from build123d import *

# Parameters (mm, degrees)
SKETCH1_R           = 1
BOSS_EXTRUDE1_DEPTH = 2.95
CUT_EXTRUDE1_DEPTH  = 0.5
SKETCH3_R           = 0.75
BOSS_EXTRUDE2_DEPTH = 3
FILLET1_R           = 0.5


with BuildPart() as part:
    # Sketch1 → Boss-Extrude1 (new body, symmetric)
    with BuildSketch(Plane(origin=(0, 0, 0), x_dir=(1, 0, 0), z_dir=(0, 1, 0))):
        Polygon((-6.5, -3.1), (-5, -3.1), (-4.5, -3.6), (-2.5, -3.6), (-2, -3.1), (2, -3.1), (2.5, -3.6), (4.5, -3.6), (5, -3.1), (6.5, -3.1), (6.5, 3.1), (5.9, 3.1), (-7.417700692, 5.9), (-7.5, 5.50855802), (3.955876716, 3.1), (-6.5, 3.1), align=None)
        with Locations((3.5, -1.9)):
            Circle(SKETCH1_R, mode=Mode.SUBTRACT)
        with Locations((-3.5, -1.9)):
            Circle(SKETCH1_R, mode=Mode.SUBTRACT)
    extrude(amount=BOSS_EXTRUDE1_DEPTH, both=True)

    # Sketch2 → Cut-Extrude1 (cut)
    with BuildSketch(Plane(origin=(0, 2.95, 0), x_dir=(1, 0, 0), z_dir=(0, 1, 0))):
        Polygon((5.9, 3.1), (3.955876716, 3.1), (-7.5, 5.50855802), (-7.417700692, 5.9), align=None)
    cut_extrude1 = extrude(amount=-CUT_EXTRUDE1_DEPTH, mode=Mode.SUBTRACT)

    # Mirror1: Cut-Extrude1 across plane
    add(cut_extrude1.mirror(Plane.ZX), mode=Mode.SUBTRACT)

    # Sketch3 → Boss-Extrude2 (add)
    with BuildSketch(Plane.XY.offset(3.1)):
        Circle(SKETCH3_R)
        with Locations((-3.5, 0)):
            Circle(SKETCH3_R)
        with Locations((3.5, 0)):
            Circle(SKETCH3_R)
    extrude(amount=BOSS_EXTRUDE2_DEPTH)

    # Fillet1
    fillet1_edges = [part.edges().sort_by_distance(p)[0] for p in [
        (-0.75, 0, 6.1),
        (-4.25, 0, 6.1),
        (2.75, 0, 6.1),
    ]]
    fillet(fillet1_edges, radius=FILLET1_R)


solid = part.part
Geometry: final body of the model. Coordinates: model frame, mm. A direction names the side the tool comes from. Coordinates: 2 decimals unless noted, no trailing zeros. Loops run counter-clockwise (first coordinate to the right, second up) from the corner with the lowest first, then second, coordinate; pieces in that order, holes last. Notation, with made-up numbers: (-28.5, -4.5) - (0.5, -4.5) arc R29 ccw to (0.5, 32.5) - close; hole circle Ø8 at (26, -19). An arc over 180 degrees is marked (long way). Put each result on its own line as item: value. Start each with the question number.
Q1. Set-up query: faces 4 (the cylindrical face through (2.75, 0.03, 4.59)), 5 (the flat face through (-1.3, -2.45, -4.4)), 6 (the flat face through (-6.5, 0, 0)), 7 (the flat face through (-1.85, 0.03, -4.32)). Return all of +Z, -Z, +X, -X, +Y, -Y with unobstructed straight access to the full face (end or side cutting, diameter ignored); none if empty.
Q2. Cut plane C-C, the plane y = -2.1. Return loops of the section in (x, z), and give its area (3 significant figures).
Q3. Cut plane B-B, the plane x = -1.5. Return loops of the section in (y, z), and give its area (3 significant figures).
Q4. Cut plane D-D, the plane z = -2.5. Return loops of the section in (x, y).
Q5. Cut plane A-A, the plane z = 1.9. Return loops of the section in (x, y), and give its area (3 significant figures).
Q6. Line query: line 1 (X direction, y = 0.55, z = 1.9); line 2 (Z direction, x = -3.5, y = -1.7); line 3 (Z direction, x = -4.25, y = 1.05). Output: solid intervals per line, ascending.
Q7. Pull-direction query (X, two-part tool) for faces 1 (the cylindrical face through (-4.25, 0.03, 4.59)), 2 (the flat face through (-0.67, 0.03, -4.48)), 3 (the flat face through (0, 2.95, -1)); classes: released by +X, released by -X, zero draft, split by the parting line, or undercut.
Q8. Pin query (flat end, axial travel): pin 1 Ø1.5 at (x, y) = (4.5, -1.5) entering from -Z; pin 2 Ø1.5 at (x, y) = (-2, -1) entering from -Z; pin 3 Ø1.2 at (x, y) = (6, 0.5) entering from +Z; pin 4 Ø0.8 at (x, z) = (1.5, -4.5) entering from +Y. Return the tip coordinate at first contact, or that it passes through.
Filled sheet:
1. face 4: +Z
1. face 5: -Z, +X, -X, -Y
1. face 6: +Z, -X, +Y, -Y
1. face 7: -X, +Y, -Y
2. outline: (-7.5, -5.51) - (-7.42, -5.9) - (5.9, -3.1) - (6.5, -3.1) - (6.5, 3.1) - (5, 3.1) - (4.5, 3.6) - (2.5, 3.6) - (2, 3.1) - (-2, 3.1) - (-2.5, 3.6) - (-4.5, 3.6) - (-5, 3.1) - (-6.5, 3.1) - (-6.5, -3.1) - (3.96, -3.1) - close; hole circle Ø2 at (-3.5, 1.9); hole circle Ø2 at (3.5, 1.9)
2. area: 81.9 mm²
3. outline: (-2.95, -3.1) - (2.95, -3.1) - (2.95, 3.1) - (-2.95, 3.1) - close; (-2.45, -4.66) - (2.45, -4.66) - (2.45, -4.25) - (-2.45, -4.25) - close
3. area: 38.6 mm²
4. outline: (-6.5, -2.95) - (6.5, -2.95) - (6.5, 2.95) - (-6.5, 2.95) - close
5. outline: (-6.5, -2.95) - (-4.5, -2.95) - (-4.5, 2.95) - (-6.5, 2.95) - close; (-2.5, -2.95) - (2.5, -2.95) - (2.5, 2.95) - (-2.5, 2.95) - close; (4.5, -2.95) - (6.5, -2.95) - (6.5, 2.95) - (4.5, 2.95) - close
5. area: 53.1 mm²
6. line 1: -6.5 to -4.5, -2.5 to 2.5, 4.5 to 6.5
6. line 2: -5.08 to -4.67, -3.1 to 0.9, 2.9 to 3.6
6. line 3: -5.23 to -4.83, -3.1 to 1.24, 2.56 to 3.6
7. face 1: undercut
7. face 2: released by +X
7. face 3: zero draft
8. pin 1: z = -3.55
8. pin 2: z = -4.92
8. pin 3: z = 3.1
8. pin 4: through
